Here's how the part is built. I have some questions about the finished solid (model axes, mm). Face numbers are marked on the shaded views. A direction names the side the tool comes from. Give positions to 0.01 mm unless a question says otherwise; leave off trailing zeros. Write each question's results on one line, items separated by ' | '. Start each with the question number.
Item 1: Please list where these lines run through material, in increasing order: line 1 along Y through (x, z) = (0, 6) (3 decimals); line 2 along X through (y, z) = (8.5, 9); line 3 along X through (y, z) = (8.25, 1.5).
Item 2: We'd pull the mould along X, two halves only. Please class the marked faces 1, 2, 3 and 4: +X half, -X half, draft (parallel to the pull), parting line (faces both ways), or undercut.
Item 3: Will these pins go through, and if not, where does the flat tip stop? P1, Ø2, axis at y = 7, z = 5, coming from the -X side; P2, Ø2, axis at y = -6.5, z = 5.5, coming from the +X side; P3, Ø3, axis at y = 3, z = 4, coming from the +X side.
Item 4: Which directions (+Z, -Z, +X, -X, +Y, -Y) give clear straight access to the entire face, cutting with the end or side of a thin tool? Please do the marked faces 5, 6, 7, 8 and 9.
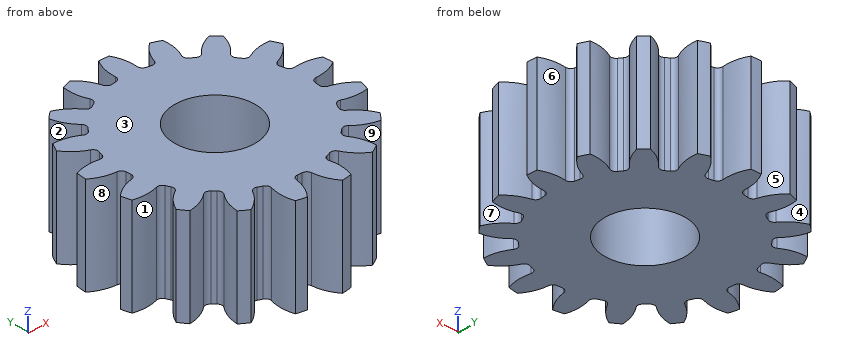
```python
from build123d import *

# Parameters (mm, degrees)
SKETCH3_R         = 12.065
GEARBODY_DEPTH    = 9.652
TOOTHCUT_DEPTH    = 10.652
CIRPATTERN1_COUNT = 17
BOREDIA_R         = 3.9624
BORE_DEPTH        = 12700


with BuildPart() as part:
    # Sketch3 → gearBody (new body)
    with BuildSketch(Plane.XY):
        Circle(SKETCH3_R)
    extrude(amount=GEARBODY_DEPTH)

    # Sketch2 → toothCut (cut, through all)
    with BuildSketch(Plane.XY):
        with BuildLine():
            ThreePointArc((9.142823661, -1.191999807), (9.169284766, -0.967628503), (9.19024048, -0.742676218))
            ThreePointArc((9.19024048, -0.742676218), (9.348086694, -0.417154866), (9.684376414, -0.283780197))
            ThreePointArc((9.684376414, -0.283780197), (11.669443263, 0.21905505), (13.194238308, 1.585925107))
            ThreePointArc((13.194238308, 1.585925107), (13.215824396, -1.39465713), (12.572564615, -4.305078625))
            ThreePointArc((12.572564615, -4.305078625), (11.366669508, -2.650040659), (9.530287729, -1.743930488))
            ThreePointArc((9.530287729, -1.743930488), (9.229245497, -1.543298603), (9.142823661, -1.191999807))
        make_face()
    toothcut = extrude(amount=TOOTHCUT_DEPTH, mode=Mode.SUBTRACT)

    # CirPattern1: toothCut ×17 about axis
    cirpattern1_axis = Axis((0, 0, 0), (0, 0, 1))
    for i in range(1, CIRPATTERN1_COUNT):
        add(toothcut.rotate(cirpattern1_axis, i * 360 / CIRPATTERN1_COUNT), mode=Mode.SUBTRACT)

    # boreDia → bore (cut, symmetric)
    with BuildSketch(Plane.XY):
        Circle(BOREDIA_R)
    extrude(amount=BORE_DEPTH, both=True, mode=Mode.SUBTRACT)


solid = part.part
```
Checked values:
1) line 1: y = -9.22 to -3.962, 3.962 to 12.065 | line 2: x = -8.35 to -6.17, -4.31 to 4.55, 6.59 to 8.56 | line 3: x = -8.27 to -5.91, -4.35 to 4.53, 6.28 to 8.55
2) face 1: undercut | face 2: -X half | face 3: draft | face 4: undercut
3) P1: stops at x = -8.18 | P2: stops at x = 9.84 | P3: stops at x = 11.9
4) face 5: +Z, -Z, +Y | face 6: +Z, -Z | face 7: +Z, -Z, +X | face 8: +Z, -Z, -X | face 9: +Z, -Z, -Y
